Here's how the part is built. I have some questions about the finished solid (model axes, mm). A direction names the side the tool comes from. Coordinates: 2 decimals unless noted, no trailing zeros. Loops run counter-clockwise (first coordinate to the right, second up) from the corner with the lowest first, then second, coordinate; pieces in that order, holes last. Notation, with made-up numbers: (18.25, 13) -> (45.25, 13) arc R25 cw to (45.25, 49) -> close; hole circle Ø9 at (80.5, 33.25). An arc over 180 degrees is marked (long way). Answer as a JSON object with one key per item and string values. Group by question number.
1) If we mould it in two halves opening along X, with no side actions, what happens to faces 1 (the flat face through (319, 0, 4.801)), 2 (the cylindrical face through (327.372, -3.905, 5.885)), 3 (the cylindrical face through (336.56, 0.18, 5.92)), 4 (the cylindrical face through (-29.536, 0.216, 0.028))? For each: +X half, -X half, draft (parallel to the pull), parting line (faces both ways), or undercut.
2) I need wall thicknesses on probe 1 along X at (y, z) = (0, -5.45); probe 2 along X at (y, z) = (-6, 12); probe 3 along X at (y, z) = (-6.5, -10.75). Which ranges of each line are inside material? Lowest first, please. Write a range as [from, to].
3) I want a section at A-A (y = 0). Count the separate pieces of the cut face and the enclosed holes in it, then the cut area to 3 significant figures.
4) I'm going to push flat-ended pins straight in: pin 1 (12.5 mm diameter, centred on y = 5.5, z = -6.5, fed in from -X); pin 2 (13.5 mm diameter, centred on y = 5.5, z = 0.5, fed in from +X); pin 3 (8 mm diameter, centred on x = 77.5, y = -8.5, fed in from +Z). Where does each tip first touch, or does it pass through?
5) Which directions (+Z, -Z, +X, -X, +Y, -Y) give clear straight access to the entire face, cutting with the end or side of a thin tool? Please do faces 5 (the flat face through (319, 0, -4.801)), 6 (the flat face through (319, 0, 7)), 7 (the flat face through (304, -9.1, -9.1)), 8 (the flat face through (-12, 0, 2)).
6) I want a section at B-B (x = 3). Write out the boundary of the cut face in (y, z).
```python
from build123d import *

# Parameters (mm, degrees)
SKETCH1_R               = 12.7
EXTRUDE1_DEPTH          = 304
SKETCH2_R               = 5
EXTRUDE2_DEPTH          = 2
SKETCH3_R               = 13.7
EXTRUDE3_DEPTH          = 4
SKETCH4_R               = 4
EXTRUDE4_DEPTH          = 7
SKETCH5_W               = 51.727972269
SKETCH5_H               = 9.602426348
CUT_EXTRUDE1_DEPTH      = 14.7
CUT_EXTRUDE1_DEPTH_BACK = 14.7


with BuildPart() as part:
    # Sketch1 → Extrude1 (new body)
    with BuildSketch(Plane(origin=(0, 0, 0), x_dir=(0, 0, -1), z_dir=(1, 0, 0))):
        Circle(SKETCH1_R)
    extrude(amount=EXTRUDE1_DEPTH)

    # Sketch2 → Extrude2 (add, symmetric)
    with BuildSketch(Plane.XY):
        with BuildLine():
            Line((0, 9.805687548), (-19.733094472, 9.805687548))
            ThreePointArc((-19.733094472, 9.805687548), (-29.53878202, 0), (-19.733094472, -9.805687548))
            Line((-19.733094472, -9.805687548), (0, -9.805687548))
            Line((0, -9.805687548), (0, 9.805687548))
        make_face()
        with Locations((-19.733094472, 0)):
            Circle(SKETCH2_R, mode=Mode.SUBTRACT)
    extrude(amount=EXTRUDE2_DEPTH, both=True)

    # Sketch3 → Extrude3 (add)
    with BuildSketch(Plane(origin=(304, 0, 0), x_dir=(0, 0, -1), z_dir=(1, 0, 0))):
        Circle(SKETCH3_R)
    extrude(amount=EXTRUDE3_DEPTH)

    # Sketch4 → Extrude4 (add, symmetric)
    with BuildSketch(Plane.XY):
        with BuildLine():
            Line((308, 8.324679236), (328.238920727, 8.324679236))
            ThreePointArc((328.238920727, 8.324679236), (336.563599963, 0), (328.238920727, -8.324679236))
            Line((328.238920727, -8.324679236), (308, -8.324679236))
            Line((308, -8.324679236), (308, 8.324679236))
        make_face()
        with Locations((328.238920727, 0)):
            Circle(SKETCH4_R, mode=Mode.SUBTRACT)
    extrude(amount=EXTRUDE4_DEPTH, both=True)

    # Sketch5 → Cut-Extrude1 (cut, two sides)
    with BuildSketch(Plane(origin=(0, 0, 0), x_dir=(1, 0, 0), z_dir=(0, 1, 0))) as cut_extrude1_sk:
        with Locations((333.863986135, 0)):
            Rectangle(SKETCH5_W, SKETCH5_H)
    extrude(amount=CUT_EXTRUDE1_DEPTH, mode=Mode.SUBTRACT)
    extrude(cut_extrude1_sk.sketch, amount=-CUT_EXTRUDE1_DEPTH_BACK, mode=Mode.SUBTRACT)


solid = part.part
```
Determined:
{
 "1": {"face 1": "draft", "face 2": "undercut", "face 3": "+X half", "face 4": "-X half"},
 "2": {"probe 1": "[0, 324.24], [332.24, 336.56]", "probe 2": "[304, 308]", "probe 3": "[0, 308]"},
 "3": {"separate pieces": "4", "enclosed holes": "0", "area": "8,000 mm^2"},
 "4": {"pin 1": "x = -29.47", "pin 2": "x = 336.56", "pin 3": "z = 11.88"},
 "5": {"face 5": "+X, +Y, -Y", "face 6": "+Z, +X, +Y, -Y", "face 7": "-X", "face 8": "+Z, -X, +Y, -Y"},
 "6": {"outline": "circle Ø25.4 at (0, 0)"}
}
